Autodesk Inventor part; units mm, degrees
ref_plane "YZ Plane" through (0, 0, 0) normal (1, 0, 0) x (0, 1, 0)
ref_plane "XZ Plane" through (0, 0, 0) normal (0, 1, 0) x (-1, 0, 0)
ref_plane "XY Plane" through (0, 0, 0) normal (0, 0, 1) x (1, 0, 0)
sketch "Sketch1" plane through (0, 0, 0) normal (0, 0, 1) x (1, 0, 0)
  line L0 (-10.25, -10.25) -> (10.25, -10.25)
  line L1 (10.25, -10.25) -> (10.25, 10.25)
  line L2 (10.25, 10.25) -> (-10.25, 10.25)
  line L3 (-10.25, 10.25) -> (-10.25, -10.25)
  line L4 (-10.25, -10.25) -> (10.25, 10.25) construction
  line L5 (10.25, -10.25) -> (-10.25, 10.25) construction
  circle A0 centre (-11, 0) radius 3.175
  arc A1 (-15.8923, 1.687) -> (-15.8923, -1.687) centre (-11, 0) ccw
  line L6 (-12.25, 12.25) -> (12.25, 12.25)
  line L7 (12.25, 12.25) -> (12.25, -12.25)
  line L8 (12.25, -12.25) -> (-12.25, -12.25)
  line L9 (-15.8923, 1.687) -> (-12.25, 12.25)
  line L10 (-15.8923, -1.687) -> (-12.25, -12.25)
  point P0 (0, 0)
  point P1 (0, 0)
  point P2 (-10.25, -3.0851)
  point P3 (-10.25, 3.0851)
  dimension "d0" = 20.5
  dimension "d1" = 20.5
  dimension "d3" = 6.35
  dimension "d4" = 11
  dimension "d5" = 2
  dimension "d6" = 2
  dimension "d7" = 2
  dimension "d8" = 2
  dimension "d10" = 2
  dimension "d11" = 2
extrude "Extrusion1" add sketch "Sketch1" against normal blind 5 contours L3 A0 L2 L1 L0 | A0 L3 | L3 A0 | L9 L6 L7 L8 L10 A1
extrude "Extrusion2" cut sketch "Sketch1" against normal blind 3 contours L3 A0 L2 L1 L0 | A0 L3 | L3 A0
sketch "Sketch2" plane through (0, 0, -3) normal (0, 0, 1) x (1, 0, 0)
  circle A0 centre (0, 0) radius 2.6
  dimension "d16" = 5.2
extrude "Extrusion3" cut sketch "Sketch2" against normal blind 10
fillet "Fillet1" radius 2 6 edges at (-10.25, 3.0851, -1.5) (-10.25, -3.0851, -1.5) (12.25, 12.25, -2.5) (12.25, -12.25, -2.5) (-12.25, 12.25, -2.5) (-12.25, -12.25, -2.5)
chamfer "Chamfer1" distance 0.75 angle 45 8 edges at (-10.25, 7.6359, 0) (-10.6742, 3.7901, 0) (-14.175, 0, 0) (-10.6742, -3.7901, 0) (-10.25, -7.6359, 0) (0, 10.25, 0) (10.25, 0, 0) (0, -10.25, 0)
properties part number "Y-Axis_Extrusion_Cap_LM3040" material "ABS Plastic"
Verification items for the finished model (mm, model axes). A direction names the side the tool comes from. Coordinates: 2 decimals unless noted, no trailing zeros. Loops run counter-clockwise (first coordinate to the right, second up) from the corner with the lowest first, then second, coordinate; pieces in that order, holes last. Notation, with made-up numbers: (-16, 21.25) -> (7, 21.25) arc R29 cw to (7, 54.25) -> close; hole circle Ø11 at (57, 6). An arc over 180 degrees is marked (long way). Answer as CSV lines item,"result".
1) Tool access check on faces 1 (the flat face through (0, 12.25, -2)), 2 (the flat face through (10.25, 0, -2)). Record the directions out of +Z, -Z, +X, -X, +Y, -Y that give a thin tool (end or side, any length) a straight path to the whole face; none if there is none.
Found:
face 1,"+Z, -Z, +X, -X, +Y"
face 2,"+Z"
2) Thickness scan on L1, parallel to Y at x = 1.75, z = -1.3; L2, parallel to Y at x = 0, z = -4.3; L3, parallel to Z at x = -13.5, y = -1.25. Record the ranges inside material, lowest first. Write a range as from..to.
Found:
L1,"y = -12.25..-10.25, 10.25..12.25"
L2,"y = -12.25..-2.6, 2.6..12.25"
L3,"z = -5..-3"
3) Cross-section at D-D, the plane x = 8.5. Record the cut outline in (y, z), then the cut area to 3 significant figures.
Found:
outline,"(-12.25, -5) -> (12.25, -5) -> (12.25, 0) -> (11, 0) -> (10.25, -0.75) -> (10.25, -3) -> (-10.25, -3) -> (-10.25, -0.75) -> (-11, 0) -> (-12.25, 0) -> close"
area,"60.4 mm2"
4) Cross-section at A-A, the plane y = 0. Record the cut outline in (x, z) (3 decimals), then the cut area to 3 significant figures.
Found:
outline,"(-16.175, -5) -> (-2.6, -5) -> (-2.6, -3) -> (-14.175, -3) -> (-14.175, -0.75) -> (-14.925, 0) -> (-16.175, 0) -> close; (2.6, -5) -> (12.25, -5) -> (12.25, 0) -> (11, 0) -> (10.25, -0.75) -> (10.25, -3) -> (2.6, -3) -> close"
area,"57.9 mm2"
5) Cross-section at B-B, the plane x = 0. Record the cut outline in (y, z).
Found:
outline,"(-12.25, -5) -> (-2.6, -5) -> (-2.6, -3) -> (-10.25, -3) -> (-10.25, -0.75) -> (-11, 0) -> (-12.25, 0) -> close; (2.6, -5) -> (12.25, -5) -> (12.25, 0) -> (11, 0) -> (10.25, -0.75) -> (10.25, -3) -> (2.6, -3) -> close"
6) Depth check by flat-ended pin: pin 1 (2 mm diameter, centred on y = -9, z = -3, fed in from -X); pin 2 (10 mm diameter, centred on x = 0.5, y = 0.5, fed in from +Z); pin 3 (2 mm diameter, centred on y = -6.5, z = -3.5, fed in from -X); pin 4 (3 mm diameter, centred on x = 0, y = 0, fed in from +Z). Enter the tip coordinate at first touch or a pass-through.
Found:
pin 1,"stops at x = -13.72"
pin 2,"stops at z = -3"
pin 3,"stops at x = -14.58"
pin 4,"passes through"
7) Cross-section at C-C, the plane z = -2.65. Record the cut outline in (x, y) (3 decimals), then the cut area to 3 significant figures.
Found:
outline,"(-15.892, -1.687) -> (-12.715, -10.902) arc R2 ccw to (-10.824, -12.25) -> (10.25, -12.25) arc R2 ccw to (12.25, -10.25) -> (12.25, 10.25) arc R2 ccw to (10.25, 12.25) -> (-10.824, 12.25) arc R2 ccw to (-12.715, 10.902) -> (-15.892, 1.687) arc R5.175 ccw to start; hole (-11.767, -3.081) arc R2 cw to (-10.25, -5.022) -> (-10.25, -10.25) -> (10.25, -10.25) -> (10.25, 10.25) -> (-10.25, 10.25) -> (-10.25, 5.022) arc R2 cw to (-11.767, 3.081) arc R3.175 ccw to start"
area,"207 mm2"
8) Release check for a two-part mould opening along Y. For faces 3 (the cylindrical face through (11.65, 11.68, -2.54)), 4 (the flat face through (-2, 2, -3)), 5 (the flat face through (0, -12.25, -2)), 6 (the cylindrical face through (-10.686, -3.776, -1.891)) record: +Y half, -Y half, draft (parallel to the pull), parting line (faces both ways), or undercut.
Found:
face 3,"+Y half"
face 4,"undercut"
face 5,"-Y half"
face 6,"undercut"
